Input: part model. Units: mm. Frame: model coordinates. A direction names the side the tool comes from. Give positions to 0.01 mm unless a question says otherwise; leave off trailing zeros. Loops run counter-clockwise (first coordinate to the right, second up) from the corner with the lowest first, then second, coordinate; pieces in that order, holes last. Notation, with made-up numbers: (54.25, 85) - (64.25, 85) arc R9 cw to (64.25, 93) - close; hole circle Ø7 at (78, -37.75). An arc over 180 degrees is marked (long way). Answer as a JSON object with one key per item and string values. Group by question number.
(1) Section query A-A (y = -41). Return loops of the section in (x, z), plus the area to 3 significant figures.
(2) Material intervals for L1, parallel to X at y = -28, z = 47.5; L2, parallel to Z at x = -51.5, y = -38.5; L3, parallel to Y at x = -86.5, z = 14, sorted ascending.
(3) Section query D-D (x = -42.5). Return loops of the section in (y, z), plus the area to 3 significant figures.
(4) Access query for faces 1 (the flat face through (50, -100.491, 24)), 2 (the cylindrical face through (-50.089, -49.277, 16.992)). Directions: +Z, -Z, +X, -X, +Y, -Y. A direction counts if a zero-diameter tool reaches every point of the face in a straight line with its end or side. Return the directions, or none.
(5) Section query B-B (z = 42). Return loops of the section in (x, y), plus the area to 3 significant figures.
(6) Pin query (flat end, axial travel): P1, Ø4, axis at y = -58.5, z = 16, coming from the -X side. Return the tip coordinate at first contact, or that it passes through.
(7) Section query C-C (z = 31.5). Return loops of the section in (x, y), plus the area to 3 significant figures.
```python
from build123d import *

# Parameters (mm, degrees)
F0_W          = 123.634026
F0_H          = 55.977793
F1_DEPTH      = 101.6
F2_R          = 13.161447
F3_DEPTH      = 203.2
F3_DEPTH_BACK = 25.4


with BuildPart() as f1:
    # F0 (on Right) → F1 (new body)
    with BuildSketch(Plane.YZ):
        with Locations((-38.673699, 24.787056)):
            Rectangle(F0_W, F0_H)
    extrude(amount=F1_DEPTH)

    # F2 (on face) → F3 (join, two sides)
    with BuildSketch(Plane.YZ.offset(101.6)) as f3_sk:
        with Locations((-38.832705, 25.00103)):
            Circle(F2_R)
    extrude(amount=-F3_DEPTH)
    extrude(f3_sk.sketch, amount=-F3_DEPTH_BACK)


solid = f1.part
```
Recorded:
{
 "1": {"outline": "(-101.6, 12.02) - (0, 12.02) - (0, -3.2) - (101.6, -3.2) - (101.6, 52.78) - (0, 52.78) - (0, 37.98) - (-101.6, 37.98) - close", "area": "8,330 mm^2"},
 "2": {"L1": "x = 0 to 101.6", "L2": "z = 11.84 to 38.16", "L3": "y = -46.06 to -31.61"},
 "3": {"outline": "circle Ø26.32 at (-38.83, 25)", "area": "544 mm^2"},
 "4": {"face 1": "+Z, -Z, +X, -X, -Y", "face 2": "-X"},
 "5": {"outline": "(0, -100.49) - (101.6, -100.49) - (101.6, 23.14) - (0, 23.14) - close", "area": "12,600 mm^2"},
 "6": {"P1": "stops at x = 0"},
 "7": {"outline": "(-101.6, -50.28) - (0, -50.28) - (0, -100.49) - (101.6, -100.49) - (101.6, 23.14) - (0, 23.14) - (0, -27.39) - (-101.6, -27.39) - close", "area": "14,900 mm^2"}
}
